Geometry: final body of the model. Coordinates: model frame, mm. A direction names the side the tool comes from. Give positions to 0.01 mm unless a question says otherwise; leave off trailing zeros. Write each loop counter-clockwise with the first axis right and the second up, starting at its lowest first coordinate (ties: lowest second). Pieces come first, ordered by that corner, then holes. Notation, with made-up numbers: M 61.25,8 L 86.25,8 A31 cw 86.25,37 Z; hole C -13.75,-28 d11. An arc over 180 degrees is marked long. Use a Markdown table: item, result. Add a question column.
(1) Draft query along Y for faces 4 (the cylindrical face through (27.35, 28.93, -5.07)), 5 (the conical face through (-11.315, 9.614, 3.288)), 6 (the flat face through (27, 34, -4)). Return one class per face: released by +Y, released by -Y, zero draft, split by the parting line, or undercut.
(2) Pin query (flat end, axial travel): pin 1 Ø3 at (x, z) = (-25.5, -3.5) entering from +Y; pin 2 Ø7 at (x, y) = (-11.69, -6.75) entering from +Z; pin 3 Ø2.5 at (y, z) = (-30.5, -5.5) entering from +X. Return the tip coordinate at first contact, or that it passes through.
(3) Reachability of faces 1 (the flat face through (-34, 28, -5)), 2 (the flat face through (34, -28, -5)), 3 (the flat face through (-29, 24, -3)) from +Z, -Z, +X, -X, +Y, -Y: full face, straight path, thin tool, end or side. Return the list, or none.
(4) Cut plane D-D (z = -5). State how many separate pieces and enclosed holes the cut face has, plus the area to 3 significant figures.
(5) Cut plane C-C (y = 29). Output: boundary loops of the cut face in (x, z), plus the area to 3 significant figures.
(6) Cut plane B-B (x = 0). Output: boundary loops of the cut face in (y, z).
(7) Cut plane A-A (y = 6.75). Output: boundary loops of the cut face in (x, z), plus the area to 3 significant figures.
(8) Material intervals for L1, parallel to Y at x = 0, z = 1.8; L2, parallel to Z at x = -29, y = -31.75; L3, parallel to Y at x = -10, z = 2, sorted ascending.
```python
from build123d import *

# Parameters (mm, degrees)
SKETCH_1_W                   = 80
SKETCH_1_H                   = 80
EXTRUDE_1_DEPTH              = 6
SKETCH_11_W                  = 10
SKETCH_11_H                  = 10
EXTRUDE_3_DEPTH              = 10
HOLE_WIZARD_M4_2_D           = 3.3
HOLE_WIZARD_M4_2_DEPTH       = 68
HOLE_WIZARD_M5_1_D           = 5.5
HOLE_WIZARD_M5_1_DEPTH       = 6
HOLE_WIZARD_M5_1_CSINK_D     = 11.2
HOLE_WIZARD_M5_1_CSINK_ANGLE = 90
MIRROR_2_COPY_1_SKETCH_W     = 10
MIRROR_2_COPY_1_SKETCH_H     = 10
MIRROR_2_COPY_1_DEPTH        = 10
MIRROR_2_COPY_2_D            = 3.3
MIRROR_2_COPY_2_DEPTH        = 68
CHAMFER_1_SIZE               = 1


with BuildPart() as part:
    # 스케치1 → 보스-돌출1 (new body)
    with BuildSketch(Plane.XY):
        Rectangle(SKETCH_1_W, SKETCH_1_H)
    extrude(amount=EXTRUDE_1_DEPTH)

    # 스케치11 → 보스-돌출3 (add)
    with BuildSketch(Plane(origin=(0, 0, 0), x_dir=(-1, 0, 0), z_dir=(0, 0, -1))):
        with Locations((29, 29)):
            Rectangle(SKETCH_11_W, SKETCH_11_H)
    extrude_3 = extrude(amount=EXTRUDE_3_DEPTH)

    # M4 나사 구멍2
    with Locations(Plane(origin=(0, 34, 0), x_dir=(1, 0, 0), z_dir=(0, 1, 0))):
        with Locations((-29, 5)):
            hole_wizard_m4_2 = Hole(HOLE_WIZARD_M4_2_D / 2, depth=HOLE_WIZARD_M4_2_DEPTH)

    # M5 육각 소켓 접시 머리 캡 나사용 카운터싱크1
    with Locations(Plane.XY.offset(6)):
        with Locations((-11.691342951, -6.75), (0, -13.5), (11.691342951, -6.75), (11.691342951, 6.75), (0, 13.5), (-11.691342951, 6.75)):
            CounterSinkHole(HOLE_WIZARD_M5_1_D / 2, HOLE_WIZARD_M5_1_CSINK_D / 2, depth=HOLE_WIZARD_M5_1_DEPTH, counter_sink_angle=HOLE_WIZARD_M5_1_CSINK_ANGLE)

    # 대칭 복사1: 보스-돌출3, M4 나사 구멍2 across plane
    add(extrude_3.mirror(Plane(origin=(0, 0, 0), x_dir=(0, 0, 1), z_dir=(1, 0, 0))))
    add(hole_wizard_m4_2.mirror(Plane(origin=(0, 0, 0), x_dir=(0, 0, 1), z_dir=(1, 0, 0))), mode=Mode.SUBTRACT)

    # 대칭 복사2: 보스-돌출3, M4 나사 구멍2 across plane
    add(extrude_3.mirror(Plane.ZX))
    add(hole_wizard_m4_2.mirror(Plane.ZX), mode=Mode.SUBTRACT)

    # 대칭 복사2 copy 1 sketch → 대칭 복사2 copy 1 (add)
    with BuildSketch(Plane(origin=(0, 0, 0), x_dir=(1, 0, 0), z_dir=(0, 0, -1))):
        with Locations((29, 29)):
            Rectangle(MIRROR_2_COPY_1_SKETCH_W, MIRROR_2_COPY_1_SKETCH_H)
    extrude(amount=MIRROR_2_COPY_1_DEPTH)

    # 대칭 복사2 copy 2
    with Locations(Plane(origin=(0, -34, 0), x_dir=(-1, 0, 0), z_dir=(0, -1, 0))):
        with Locations((-29, 5)):
            Hole(MIRROR_2_COPY_2_D / 2, depth=MIRROR_2_COPY_2_DEPTH)

    # 모따기1
    chamfer_1_edges = [part.edges().sort_by_distance(p)[0] for p in [
        (34, -34, -5),
        (-34, -34, -5),
        (-34, 34, -5),
        (34, 34, -5),
    ]]
    chamfer(chamfer_1_edges, length=CHAMFER_1_SIZE)


solid = part.part
```
Answer list:
| question | item | result |
|---|---|---|
| 1 | face 4 | zero draft |
| 1 | face 5 | undercut |
| 1 | face 6 | released by +Y |
| 2 | pin 1 | y = 34 |
| 2 | pin 2 | z = 3.9 |
| 2 | pin 3 | x = 34 |
| 3 | face 1 | -Z, -X, +Y, -Y |
| 3 | face 2 | -Z, +X, +Y, -Y |
| 3 | face 3 | -Z, +X, -X |
| 4 | separate pieces | 8 |
| 4 | enclosed holes | 0 |
| 4 | area | 266 mm² |
| 5 | outline | M -40,0 L -34,0 L -34,-10 L -24,-10 L -24,0 L 24,0 L 24,-10 L 34,-10 L 34,0 L 40,0 L 40,6 L -40,6 Z; hole C -29,-5 d3.3; hole C 29,-5 d3.3 |
| 5 | area | 663 mm² |
| 6 | outline | M -40,0 L -16.25,0 L -16.25,3.15 L -19.1,6 L -40,6 Z; M -10.75,0 L 10.75,0 L 10.75,3.15 L 7.9,6 L -7.9,6 L -10.75,3.15 Z; M 16.25,0 L 40,0 L 40,6 L 19.1,6 L 16.25,3.15 Z |
| 7 | outline | M -40,0 L -14.44,0 L -14.44,3.15 L -17.29,6 L -40,6 Z; M -8.94,0 L 8.94,0 L 8.94,3.15 L 6.09,6 L -6.09,6 L -8.94,3.15 Z; M 14.44,0 L 40,0 L 40,6 L 17.29,6 L 14.44,3.15 Z |
| 7 | area | 398 mm² |
| 8 | L1 | -40 to -16.25, -10.75 to 10.75, 16.25 to 40 |
| 8 | L2 | -10 to -6.65, -3.35 to 6 |
| 8 | L3 | -40 to -8.92, -4.58 to 4.58, 8.92 to 40 |
